from build123d import *

# Parameters (mm, degrees)
SKETCH1_R              = 2.5
EXTRUDE_1_DEPTH        = 260
HOLE_WIZARD_M6_1_D     = 5
HOLE_WIZARD_M6_1_DEPTH = 20
HOLE_WIZARD_M6_1_TIP   = 1.502151548
HOLE_WIZARD_M6_2_D     = 5
HOLE_WIZARD_M6_2_DEPTH = 20
HOLE_WIZARD_M6_2_TIP   = 1.502151548


with BuildPart() as part:
    # Sketch1 → 凸台-拉伸1 (new body)
    with BuildSketch(Plane.XY):
        with BuildLine():
            Line((-6, -15), (-3.25, -15))
            Line((-3.25, -15), (-3.25, -13))
            Line((-3.25, -13), (-5, -13))
            Line((-5, -13), (-5, -6))
            Line((-5, -6), (-3.25, -6))
            Line((-3.25, -6), (-3.25, -4))
            Line((-3.25, -4), (3.25, -4))
            Line((3.25, -4), (3.25, -6))
            Line((3.25, -6), (5, -6))
            Line((5, -6), (5, -13))
            Line((5, -13), (3.25, -13))
            Line((3.25, -13), (3.25, -15))
            Line((3.25, -15), (6, -15))
            ThreePointArc((6, -15), (7.060660172, -14.560660172), (7.5, -13.5))
            Line((7.5, -13.5), (7.5, 13.5))
            ThreePointArc((7.5, 13.5), (7.060660172, 14.560660172), (6, 15))
            Line((6, 15), (3.25, 15))
            Line((3.25, 15), (3.25, 13))
            Line((3.25, 13), (5, 13))
            Line((5, 13), (5, 6))
            Line((5, 6), (3.25, 6))
            Line((3.25, 6), (3.25, 4))
            Line((3.25, 4), (-3.25, 4))
            Line((-3.25, 4), (-3.25, 6))
            Line((-3.25, 6), (-5, 6))
            Line((-5, 6), (-5, 13))
            Line((-5, 13), (-3.25, 13))
            Line((-3.25, 13), (-3.25, 15))
            Line((-3.25, 15), (-6, 15))
            ThreePointArc((-6, 15), (-7.060660172, 14.560660172), (-7.5, 13.5))
            Line((-7.5, 13.5), (-7.5, -13.5))
            ThreePointArc((-7.5, -13.5), (-7.060660172, -14.560660172), (-6, -15))
        make_face()
        Circle(SKETCH1_R, mode=Mode.SUBTRACT)
    extrude(amount=EXTRUDE_1_DEPTH)

    # M6 螺纹孔1
    with Locations(Plane.XY.offset(260)):
        with Locations((0, 0)):
            Hole(HOLE_WIZARD_M6_1_D / 2, depth=HOLE_WIZARD_M6_1_DEPTH)
            with Locations((0, 0, -(HOLE_WIZARD_M6_1_DEPTH + HOLE_WIZARD_M6_1_TIP / 2))):  # 118° drill point
                Cone(0, HOLE_WIZARD_M6_1_D / 2, HOLE_WIZARD_M6_1_TIP, mode=Mode.SUBTRACT)

    # M6 螺纹孔2
    with Locations(Plane(origin=(0, 0, 0), x_dir=(-1, 0, 0), z_dir=(0, 0, -1))):
        with Locations((0, 0)):
            Hole(HOLE_WIZARD_M6_2_D / 2, depth=HOLE_WIZARD_M6_2_DEPTH)
            with Locations((0, 0, -(HOLE_WIZARD_M6_2_DEPTH + HOLE_WIZARD_M6_2_TIP / 2))):  # 118° drill point
                Cone(0, HOLE_WIZARD_M6_2_D / 2, HOLE_WIZARD_M6_2_TIP, mode=Mode.SUBTRACT)


solid = part.part
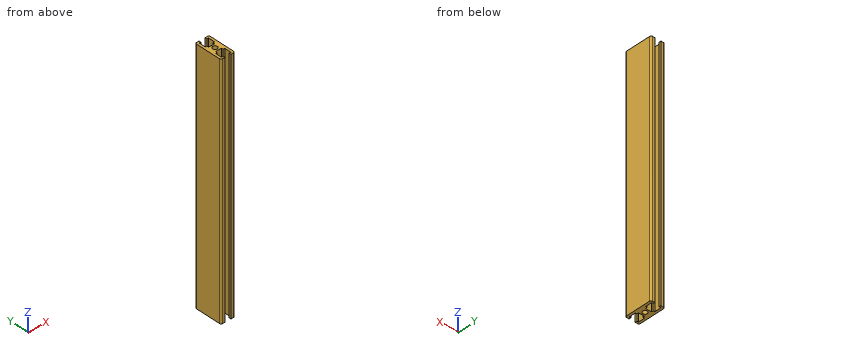
The listing builds one solid part. Answer for the finished solid, in the listing's coordinates (mm). Round coordinates to 2 decimals unless told otherwise and drop trailing zeros. Loops run counter-clockwise (first coordinate to the right, second up) from the corner with the lowest first, then second, coordinate; pieces in that order, holes last. Notation, with made-up numbers: M 45,-17.5 L 70,-17.5 A8 cw 70,-10.5 Z; hole C 17,80.5 d11. An arc over 180 degrees is marked long. Write each question's results on one line, items separated by ' | '. Start each with the question number.
1) Find section A-A on y = 0. Write down the section's boundary in (x, z).
2) Each of these flat-tipped pins is pushed along its axis until it touches: pin 1 (6 mm diameter, centred on x = 0.5, y = -6, fed in from -Z); pin 2 (4 mm diameter, centred on x = -1, y = 10.5, fed in from -Z); pin 3 (5 mm diameter, centred on x = -0.5, z = 138, fed in from +Y); pin 4 (3 mm diameter, centred on x = -0.5, z = 153.5, fed in from -Y). Where does it stop, or does it pass through?
3) Straight lines are drawn through the part: probe 1 along Y at (x, z) = (-0.5, 131); probe 2 along X at (y, z) = (5.5, 24.5); probe 3 along Y at (x, z) = (0, 88). For each, find the intervals that lie inside material, in ascending order.
4) Find section B-B on x = 0. Write down the section's boundary in (y, z).
Final values:
1) outline: M -7.5,0 L -2.5,0 L -2.5,260 L -7.5,260 Z; M 2.5,0 L 7.5,0 L 7.5,260 L 2.5,260 Z
2) pin 1: z = 0 | pin 2: through | pin 3: y = 4 | pin 4: y = -4
3) probe 1: -4 to -2.45, 2.45 to 4 | probe 2: -7.5 to -3.25, 3.25 to 7.5 | probe 3: -4 to -2.5, 2.5 to 4
4) outline: M -4,0 L -2.5,0 L -2.5,260 L -4,260 Z; M 2.5,0 L 4,0 L 4,260 L 2.5,260 Z
